Can you work these out from the model? Positions are in its coordinate system, mm. A direction names the side the tool comes from. Round coordinates to 2 decimals unless told otherwise and drop trailing zeros. Write each loop counter-clockwise with the first axis right and the second up, starting at its lowest first coordinate (ties: lowest second). Pieces come first, ordered by that corner, then holes. Notation, with made-up numbers: M -3.75,55 L 52.25,55 A27 ccw 52.25,79 Z; hole C 65.25,76.5 d1. An arc over 180 degrees is marked long. Answer in a Markdown table with one row per item. Add a question column.
(1) Suppose I cut it at A-A, the plane z = 0. Write out the boundary of the cut face in (x, y), then the cut area to 3 significant figures.
(2) If I drill on probe 1 along X at (y, z) = (5.5, 0); probe 2 along Y at (x, z) = (21.5, 2); probe 3 along X at (y, z) = (-2.5, -224.5), over which ranges is the centre line in solid material (lowest first)?
(3) For faces 1 (the face through (-34.506, -10, -220)), 2 (the face through (-65, -20, -220)), 3 (the face through (-94.506, -10, -220)), which set-ups out of +Z, -Z, +X, -X, +Y, -Y let a thin tool reach every point of the face, with its end or its side?
(4) Suppose I cut it at B-B, the plane x = -290. Write out the boundary of the cut face in (y, z), then the cut area to 3 significant figures.
(5) If we mould it in two halves opening along Z, with no side actions, what happens to faces 4 (the face through (-65, -10, -190)), 5 (the face through (315.476, 9.86, -4.336)), 6 (the face through (400, 10, 0))? For each: released by +Z, released by -Z, zero draft, split by the parting line, or undercut.
(6) I'm going to push flat-ended pins straight in: pin 1 (16 mm diameter, centred on y = -10, z = -231, fed in from -X); pin 2 (16 mm diameter, centred on y = -13, z = -214, fed in from +X); pin 3 (10 mm diameter, centred on x = -71.5, y = -9.5, fed in from +Z). Where does each tip first touch, or does it pass through?
from build123d import *

# Parameters (mm, degrees)
SKETCH1_R           = 20
BOSS_EXTRUDE1_DEPTH = 20
SKETCH2_W           = 60
SKETCH2_H           = 60
BOSS_EXTRUDE2_DEPTH = 20
SKETCH3_R           = 5
CUT_EXTRUDE1_DEPTH  = 20


with BuildPart() as part:
    # Sketch1 → Boss-Extrude1 (new body)
    with BuildSketch(Plane(origin=(0, 0, 0), x_dir=(1, 0, 0), z_dir=(0, 1, 0))):
        with BuildLine():
            Line((-300, 250), (270.987668093, 250))
            add(Edge.make_bspline(
                [(270.987668093, 250), (197.722942543, 110.46504325), (360.729994598, 99.497758331), (400, 31.506674192)],
                knots=[0, 0, 0, 0, 0.79710865, 0.79710865, 0.79710865, 0.79710865], degree=3))
            Line((400, 31.506674192), (400, -31.506674192))
            add(Edge.make_bspline(
                [(270.987668093, -250), (197.722942543, -110.46504325), (360.729994598, -99.497758331), (400, -31.506674192)],
                knots=[0, 0, 0, 0, 0.79710865, 0.79710865, 0.79710865, 0.79710865], degree=3))
            Line((270.987668093, -250), (-300, -250))
            ThreePointArc((-300, -250), (-370.710678119, -220.710678119), (-400, -150))
            Line((-400, -150), (-400, 150))
            ThreePointArc((-400, 150), (-370.710678119, 220.710678119), (-300, 250))
        make_face()
        with Locations(Location((335, 0, 0), (0, 0, 270))):
            Circle(SKETCH1_R, mode=Mode.SUBTRACT)
    extrude(amount=BOSS_EXTRUDE1_DEPTH)

    # Sketch2 → Boss-Extrude2 (add)
    with BuildSketch(Plane.XZ):
        with Locations((-64.506165954, -220)):
            Rectangle(SKETCH2_W, SKETCH2_H)
    extrude(amount=BOSS_EXTRUDE2_DEPTH)

    # Sketch3 → Cut-Extrude1 (cut)
    with BuildSketch(Plane(origin=(0, 0, -250), x_dir=(-1, 0, 0), z_dir=(0, 0, -1))):
        with Locations((64.506165954, 0)):
            Circle(SKETCH3_R)
    extrude(amount=-CUT_EXTRUDE1_DEPTH, mode=Mode.SUBTRACT)


solid = part.part
Calculated:
| question | item | result |
|---|---|---|
| 1 | outline | M -400,0 L 315,0 L 315,20 L -400,20 Z; M 355,0 L 400,0 L 400,20 L 355,20 Z |
| 1 | area | 15,200 mm² |
| 2 | probe 1 | -400 to 315, 355 to 400 |
| 2 | probe 2 | 0 to 20 |
| 2 | probe 3 | -94.51 to -34.51 |
| 3 | face 1 | +Z, -Z, +X, -Y |
| 3 | face 2 | +Z, -Z, +X, -X, -Y |
| 3 | face 3 | +Z, -Z, -X, -Y |
| 4 | outline | M 0,-250 L 20,-250 L 20,250 L 0,250 Z |
| 4 | area | 10,000 mm² |
| 5 | face 4 | released by +Z |
| 5 | face 5 | undercut |
| 5 | face 6 | zero draft |
| 6 | pin 1 | x = -94.51 |
| 6 | pin 2 | x = -34.51 |
| 6 | pin 3 | z = -190 |
